from build123d import *

# Parameters (mm, degrees)
SKETCH1_R            = 8.5
BOSS_EXTRUDE1_DEPTH  = 10
FILLET2_R            = 1
M3_CLEARANCE_HOLE1_D = 3.4


with BuildPart() as part:
    # Sketch1 → Boss-Extrude1 (new body)
    with BuildSketch(Plane(origin=(0, 0, 0), x_dir=(1, 0, 0), z_dir=(0, 1, 0))):
        with Locations(Location((0, 0, 0), (0, 0, 270))):
            Circle(SKETCH1_R)
    extrude(amount=BOSS_EXTRUDE1_DEPTH)

    # Fillet2
    fillet2_edges = [part.edges().sort_by_distance(p)[0] for p in [
        (0, 10, -8.5),
    ]]
    fillet(fillet2_edges, radius=FILLET2_R)

    # M3 Clearance Hole1 (through all)
    with Locations(Plane(origin=(0, 10, 0), x_dir=(1, 0, 0), z_dir=(0, 1, 0))):
        with Locations((-5, 0), (5, 0)):
            Hole(M3_CLEARANCE_HOLE1_D / 2)


solid = part.part
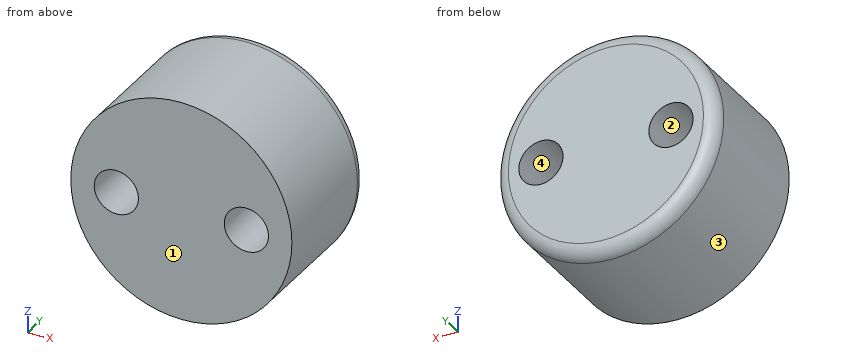
Build history of the part. All positions in model axes, mm. Face numbers are marked on the shaded views. Coordinates: 2 decimals unless noted, no trailing zeros. Order: outer loops, then holes, each group sorted by start corner. A loop starts at its lowest first (then second) coordinate and runs counter-clockwise, first axis right, second up. Notation, with made-up numbers: (39, 46) - (80, 46) arc R22 ccw to (80, 79) - close; hole circle Ø3 at (-31, 12). An arc over 180 degrees is marked (long way). Write each question's results on one line, items separated by ' | '. Start each with the question number.
Item 1: Wall check: probe 1 along X at (y, z) = (4.5, 1.5); probe 2 along Z at (x, y) = (5, 5.5); probe 3 along Z at (x, y) = (-5.25, 4.5). Give the ranges that are in metal, low to high. Write a range as [from, to].
Item 2: Band-saw the part on A-A on z = 0. Write the cut outline in (x, y).
Item 3: Band-saw the part on B-B on y = 0.75. Write the cut outline in (x, z), and give its area (3 significant figures).
Item 4: Flat gauge pins, fed straight in: pin 1 (1.5 mm diameter, centred on x = 2, y = 5.5, fed in from -Z); pin 2 (6 mm diameter, centred on y = 2, z = -4.5, fed in from -X); pin 3 (6 mm diameter, centred on y = 8.5, z = -5.5, fed in from -X). Where does each tip first touch, or does it go through?
Item 5: Mould opens along Z. For the marked faces 1, 2, 3 and 4 say: released by +Z, released by -Z, zero draft, split by the parting line, or undercut.
Item 6: Band-saw the part on C-C on y = 9.5. Write the cut outline in (x, z).
Numbers:
1) probe 1: [-8.37, -5.8], [-4.2, 4.2], [5.8, 8.37] | probe 2: [-6.87, -1.7], [1.7, 6.87] | probe 3: [-6.68, -1.68], [1.68, 6.68]
2) outline: (-8.5, 0) - (-6.7, 0) - (-6.7, 10) - (-7.5, 10) arc R1 ccw to (-8.5, 9) - close; (-3.3, 0) - (3.3, 0) - (3.3, 10) - (-3.3, 10) - close; (6.7, 0) - (8.5, 0) - (8.5, 9) arc R1 ccw to (7.5, 10) - (6.7, 10) - close
3) outline: circle Ø17 at (0, 0); hole circle Ø3.4 at (-5, 0); hole circle Ø3.4 at (5, 0) | area: 209 mm^2
4) pin 1: z = -8.41 | pin 2: x = -8.37 | pin 3: x = -8.12
5) face 1: zero draft | face 2: undercut | face 3: split by the parting line | face 4: undercut
6) outline: circle Ø16.73 at (0, 0); hole circle Ø3.4 at (-5, 0); hole circle Ø3.4 at (5, 0)
